The listing builds one solid part. Answer for the finished solid, in the listing's coordinates (mm). Face numbers are marked on the shaded views. A direction names the side the tool comes from. Round coordinates to 2 decimals unless told otherwise and drop trailing zeros. Order: outer loops, then holes, each group sorted by start corner. A loop starts at its lowest first (then second) coordinate and runs counter-clockwise, first axis right, second up. Notation, with made-up numbers: M 61,52.25 L 104,52.25 A19 cw 104,70.25 Z; hole C -35.75,27 d9. An arc over 180 degrees is marked long. Write item = value, one per line. Start each with the question number.
(1) Straight lines are drawn through the part: probe 1 along Y at (x, z) = (0, 266); probe 2 along Z at (x, y) = (-8.5, 4); probe 3 along Y at (x, z) = (55, 71). For each, find the intervals that lie inside material, in ascending order. Write a range as from..to.
(2) A cutting plane is placed at B-B, the plane x = 0. Determine the outline of the cut face in (y, z), and give its area (3 significant figures).
(3) A cutting plane is placed at A-A, the plane y = 0. Determine the outline of the cut face in (x, z), and give its area (3 significant figures).
(4) A cutting plane is placed at C-C, the plane x = -47. Determine the outline of the cut face in (y, z), and give its area (3 significant figures).
(5) Which of the six approach directions +Z, -Z, +X, -X, +Y, -Y give full straight-line access (tool end or side, diameter ignored) to the marked faces 5, 6, 7, 8 and 9?
(6) For a pull along Y with two mould halves and no side action, classify the marked faces 1, 2, 3 and 4 as released by +Y, released by -Y, zero draft, split by the parting line, or undercut.
(7) Each of these flat-tipped pins is pushed along its axis until it touches: pin 1 (9 mm diameter, centred on x = 42.5, z = 185, fed in from +Y); pin 2 (15 mm diameter, centred on x = -47.5, z = 147.5, fed in from -Y); pin 3 (10 mm diameter, centred on x = -11, z = 208, fed in from -Y). Where does it stop, or does it pass through?
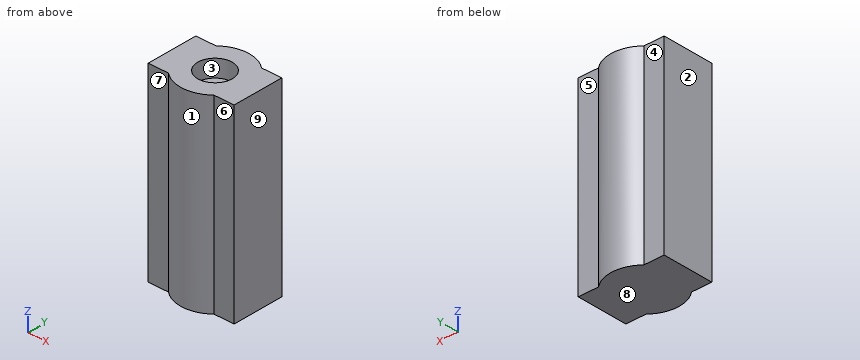
from build123d import *

# Parameters (mm, degrees)
F1_DEPTH = 254
F2_R     = 25.4
F3_DEPTH = 25.4


with BuildPart() as f1:
    # F0 (on Top) → F1 (new body)
    with BuildSketch(Plane.XY):
        with BuildLine():
            Line((-63.5, -38.1), (-33.601042, -38.1))
            ThreePointArc((-33.601042, -38.1), (0, -50.8), (33.601042, -38.1))
            Line((33.601042, -38.1), (63.5, -38.1))
            Line((63.5, -38.1), (63.5, 38.1))
            Line((63.5, 38.1), (33.601042, 38.1))
            ThreePointArc((33.601042, 38.1), (0, 50.8), (-33.601042, 38.1))
            Line((-33.601042, 38.1), (-63.5, 38.1))
            Line((-63.5, 38.1), (-63.5, -38.1))
        make_face()
    extrude(amount=F1_DEPTH)

    # F2 (on face) → F3 (join)
    with BuildSketch(Plane.XY.offset(254)):
        with BuildLine():
            ThreePointArc((33.601042, 38.1), (0, 50.8), (-33.601042, 38.1))
            Line((-33.601042, 38.1), (-63.5, 38.1))
            Line((-63.5, 38.1), (-63.5, -38.1))
            Line((-63.5, -38.1), (-33.601042, -38.1))
            ThreePointArc((-33.601042, -38.1), (0, -50.8), (33.601042, -38.1))
            Line((33.601042, -38.1), (63.5, -38.1))
            Line((63.5, -38.1), (63.5, 38.1))
            Line((63.5, 38.1), (33.601042, 38.1))
        make_face()
        Circle(F2_R, mode=Mode.SUBTRACT)
    extrude(amount=F3_DEPTH)


solid = f1.part
Reported:
q1.probe_1 = -50.8..-25.4, 25.4..50.8
q1.probe_2 = 0..254
q1.probe_3 = -38.1..38.1
q2.outline = M -50.8,0 L 50.8,0 L 50.8,279.4 L 25.4,279.4 L 25.4,254 L -25.4,254 L -25.4,279.4 L -50.8,279.4 Z
q2.area = 27,100 mm²
q3.outline = M -63.5,0 L 63.5,0 L 63.5,279.4 L 25.4,279.4 L 25.4,254 L -25.4,254 L -25.4,279.4 L -63.5,279.4 Z
q3.area = 34,200 mm²
q4.outline = M -38.1,0 L 38.1,0 L 38.1,279.4 L -38.1,279.4 Z
q4.area = 21,300 mm²
q5.face_5 = +Z, -Z, +X, +Y
q5.face_6 = +Z, -Z, +X, -Y
q5.face_7 = +Z, -Z, -X, -Y
q5.face_8 = -Z, +X, -X, +Y, -Y
q5.face_9 = +Z, -Z, +X, +Y, -Y
q6.face_1 = released by -Y
q6.face_2 = zero draft
q6.face_3 = undercut
q6.face_4 = released by +Y
q7.pin_1 = 38.1
q7.pin_2 = -38.1
q7.pin_3 = -50.44
